from build123d import *

# Parameters (mm, degrees)
BOSS_EXTRU_1_DEPTH      = 5
CONG_2_R                = 1.5
CONG_3_R                = 0.5
ESQUISSE3_W             = 2.5
ESQUISSE3_H             = 4
ENL_V_MAT_EXTRU_1_DEPTH = 1.3
ESQUISSE4_W             = 2.5
ESQUISSE4_H             = 0.3
ENL_V_MAT_EXTRU_2_DEPTH = 0.4
ESQUISSE5_W             = 2.5
ESQUISSE5_H             = 2
BOSS_EXTRU_2_DEPTH      = 0.5
CONG_4_R                = 0.3


with BuildPart() as part:
    # Esquisse2 → Boss.-Extru.1 (new body)
    with BuildSketch(Plane.XY):
        with BuildLine():
            Line((0, 0), (-3.7, 0))
            Line((-3.7, 0), (-3.7, 16.217812561))
            ThreePointArc((-3.7, 16.217812561), (-3.586649408, 16.386494959), (-3.387643104, 16.345280892))
            Line((-3.387643104, 16.345280892), (1.376192195, 11.480497264))
            Line((1.376192195, 11.480497264), (0.107236318, 4.755627118))
            Line((0.107236318, 4.755627118), (0.402033916, 4.7))
            Line((0.402033916, 4.7), (1.7, 11.578610619))
            Line((1.7, 11.578610619), (-3.173298816, 16.555177357))
            ThreePointArc((-3.173298816, 16.555177357), (-3.7, 16.664256805), (-4, 16.217812561))
            Line((-4, 16.217812561), (-4, -0.3))
            Line((-4, -0.3), (0, -0.3))
            Line((0, -0.3), (0, 0))
        make_face()
    extrude(amount=BOSS_EXTRU_1_DEPTH)

    # Congé2
    cong_2_edges = [part.edges().sort_by_distance(p)[0] for p in [
        (1.376192195, 11.480497264, 2.5),
        (1.7, 11.578610619, 2.5),
    ]]
    fillet(cong_2_edges, radius=CONG_2_R)

    # Congé3
    cong_3_edges = [part.edges().sort_by_distance(p)[0] for p in [
        (-3.7, 0, 2.5),
        (-4, -0.3, 2.5),
    ]]
    fillet(cong_3_edges, radius=CONG_3_R)

    # Esquisse3 → Enlèv. mat.-Extru.1 (cut)
    with BuildSketch(Plane.ZY.offset(4)):
        with Locations((2.5, 1.7)):
            Rectangle(ESQUISSE3_W, ESQUISSE3_H)
    extrude(amount=-ENL_V_MAT_EXTRU_1_DEPTH, mode=Mode.SUBTRACT)

    # Esquisse4 → Enlèv. mat.-Extru.2 (cut)
    with BuildSketch(Plane(origin=(0, 0, 0), x_dir=(0, 0, -1), z_dir=(1, 0, 0))):
        with Locations((-2.5, -0.15)):
            Rectangle(ESQUISSE4_W, ESQUISSE4_H)
    extrude(amount=-ENL_V_MAT_EXTRU_2_DEPTH, mode=Mode.SUBTRACT)

    # Esquisse5 → Boss.-Extru.2 (add)
    with BuildSketch(Plane(origin=(-0.4, 0, 0), x_dir=(0, 0, -1), z_dir=(1, 0, 0))):
        with Locations((-2.5, -1.3)):
            Rectangle(ESQUISSE5_W, ESQUISSE5_H)
    boss_extru_2 = extrude(amount=-BOSS_EXTRU_2_DEPTH)

    # Symétrie1: Boss.-Extru.2 across plane
    add(boss_extru_2.mirror(Plane(origin=(-1.55, 0, 0), x_dir=(0, 0, 1), z_dir=(1, 0, 0))))

    # Congé4
    cong_4_edges = [part.edges().sort_by_distance(p)[0] for p in [
        (-0.4, 0, 2.5),
        (-2.7, 0, 2.5),
        (-0.9, -0.3, 2.5),
        (-2.2, -0.3, 2.5),
    ]]
    fillet(cong_4_edges, radius=CONG_4_R)


solid = part.part
CAD build for the part. Positions are in the model's coordinates, mm. A direction names the side the tool comes from. Give positions to 0.01 mm unless a question says otherwise; leave off trailing zeros. Write each loop counter-clockwise with the first axis right and the second up, starting at its lowest first coordinate (ties: lowest second). Pieces come first, ordered by that corner, then holes. Notation, with made-up numbers: M 36.5,77.25 L 68.5,77.25 A22 ccw 68.5,109.25 Z; hole C 83,-1 d2. An arc over 180 degrees is marked long. Put each result on its own line as item: value. Start each with the question number.
(1) Band-saw the part on A-A, the plane y = -1. Write the cut outline in (x, z), and give its area (3 significant figures).
(2) Band-saw the part on C-C, the plane x = -2.9. Write the cut outline in (y, z), and give its area (3 significant figures).
(3) Mould opens along X. For faces 1 (the face through (-1.309, 14.222, 2.465)), 2 (the face through (0.97, 7.71, 2.46)), 3 (the face through (-0.9, -1, 3)), 4 (the face through (-2.7, -1, 3)) say: +X half, -X half, draft (parallel to the pull), parting line (faces both ways), or undercut.
(4) Flat gauge pins, fed straight in: pin 1 Ø0.9 at (x, y) = (-1, -1.5) entering from +Z; pin 2 Ø1.5 at (x, z) = (-1.5, 4.5) entering from +Y; pin 3 Ø0.5 at (x, y) = (-3, 1) entering from -Z; pin 4 Ø0.9 at (x, y) = (-1, -1) entering from -Z. Where does each tip first touch, or does it go through?
(5) Band-saw the part on B-B, the plane z = 2.45. Write the cut outline in (x, y).
(6) Which spindle directions (+Z, -Z, +X, -X, +Y, -Y) get a long thin tool onto all of the face, cutting with end or side? Do faces 5 (the face through (-2, 0, 2)), 6 (the face through (0.677, 7.775, 2.465)), 7 (the face through (-0.4, -1, 3)). Say none if no direction does.
(7) Band-saw the part on D-D, the plane z = 4.2. Write the cut outline in (x, y).
(8) Probe L1, parallel to X at y = 2.25, z = 0.65; L2, parallel to Y at x = -0.1, z = 4.3; L3, parallel to Y at x = -3.05, z = 4.7. List the from-to ranges inside material, lowest first.
Response values:
1. outline: M -2.7,1.25 L -2.2,1.25 L -2.2,3.75 L -2.7,3.75 Z; M -0.9,1.25 L -0.4,1.25 L -0.4,3.75 L -0.9,3.75 Z
1. area: 2.50 mm2
2. outline: M -0.3,0 L 0,0 L 0,1.25 L -0.3,1.25 Z; M -0.3,3.75 L 0,3.75 L 0,5 L -0.3,5 Z; M 15.85,0 L 16.28,0 L 16.28,5 L 15.85,5 Z
2. area: 2.89 mm2
3. face 1: undercut
3. face 2: +X half
3. face 3: undercut
3. face 4: -X half
4. pin 1: stops at z = 3.75
4. pin 2: stops at y = 15.61
4. pin 3: passes through
4. pin 4: stops at z = 1.25
5. outline: M -4,3.7 L -3.7,3.7 L -3.7,16.22 A0.18 cw -3.39,16.35 L 0.83,12.04 A1.5 cw 1.23,10.71 L 0.11,4.76 L 0.4,4.7 L 1.55,10.81 A1.5 ccw 1.15,12.14 L -3.17,16.56 A0.48 ccw -4,16.22 Z; M -2.7,-2.3 L -2.2,-2.3 L -2.2,-0.6 A0.3 cw -1.9,-0.3 L -1.2,-0.3 A0.3 cw -0.9,-0.6 L -0.9,-2.3 L -0.4,-2.3 L -0.4,-0.3 A0.3 ccw -0.7,0 L -2.4,0 A0.3 ccw -2.7,-0.3 Z
6. face 5: +Z, -Z, +X
6. face 6: +Z, -Z
6. face 7: +Z, -Z, +X, -Y
7. outline: M -4,0.2 A0.5 ccw -3.5,-0.3 L 0,-0.3 L 0,0 L -3.2,0 A0.5 cw -3.7,0.5 L -3.7,16.22 A0.18 cw -3.39,16.35 L 0.83,12.04 A1.5 cw 1.23,10.71 L 0.11,4.76 L 0.4,4.7 L 1.55,10.81 A1.5 ccw 1.15,12.14 L -3.17,16.56 A0.48 ccw -4,16.22 Z
8. L1: x = -4 to -3.7
8. L2: y = -0.3 to 0, 12.99 to 13.42
8. L3: y = -0.3 to 0, 16 to 16.43
